```python
from build123d import *

# Parameters (mm, degrees)
F0_W     = 25.4
F0_H     = 25.4
F1_DEPTH = 304.8
F2_R     = 3.175
F3_DEPTH = 50.8
F4_R     = 3.175
F5_DEPTH = 25.4
F6_R     = 3.175
F7_DEPTH = 25.4
F8_DEPTH = 12.7


with BuildPart() as f1:
    # F0 (on Top) → F1 (new body)
    with BuildSketch(Plane.XY):
        Rectangle(F0_W, F0_H)
    extrude(amount=F1_DEPTH)

    # F2 (on face) → F3 (cut)
    with BuildSketch(Plane.XZ.offset(12.7)):
        with Locations((0, 292.1)):
            Circle(F2_R)
    extrude(amount=-F3_DEPTH, mode=Mode.SUBTRACT)

    # F4 (on face) → F5 (cut)
    with BuildSketch(Plane.YZ.offset(12.7)):
        with Locations((0, 292.1)):
            Circle(F4_R)
    extrude(amount=-F5_DEPTH, mode=Mode.SUBTRACT)

    # F6 (on face) → F7 (cut)
    with BuildSketch(Plane.YZ.offset(12.7)):
        with Locations((0, 4.7888585575)):
            Circle(F6_R)
    extrude(amount=-F7_DEPTH, mode=Mode.SUBTRACT)

    # F8 (add): a face of the model
    f8_faces = [f1.faces().sort_by_distance(p)[0] for p in [
        (0, 0, 0),
    ]]
    extrude(f8_faces, amount=F8_DEPTH)


solid = f1.part
```
Model file for the job. Use its own axes, mm. Give positions to 0.01 mm unless a question says otherwise; leave off trailing zeros. Order: outer loops, then holes, each group sorted by start corner. A loop starts at its lowest first (then second) coordinate and runs counter-clockwise, first axis right, second up.
1) Mould opens along Z. For faces 1 (the flat face through (12.7, 0, 148)), 2 (the cylindrical face through (3.03, -7.85, 293.05)), 3 (the flat face through (0, 0, -12.7)) say: +Z half, -Z half, draft (parallel to the pull), parting line (faces both ways), or undercut.
2) Wall check: probe 1 along Z at (x, y) = (5.5, 0) (3 decimals); probe 2 along Z at (x, y) = (-3.5, 0.5); probe 3 along Y at (x, z) = (-7.5, 292.1) (3 decimals). Give the ranges that are in metal, low to high.
3) Saw through at A-A, the plane z = 292.1. Write the cut outline in (x, y) (3 decimals), then the cut area to 3 significant figures.
Computed:
1. face 1: draft
1. face 2: undercut
1. face 3: -Z half
2. probe 1: z = -12.7 to 1.614, 7.964 to 288.925, 295.275 to 304.8
2. probe 2: z = -12.7 to 1.65, 7.92 to 288.96, 295.24 to 304.8
2. probe 3: y = -12.7 to -3.175, 3.175 to 12.7
3. outline: (-12.7, -12.7) - (-3.175, -12.7) - (-3.175, -3.175) - (-12.7, -3.175) - close; (-12.7, 3.175) - (-3.175, 3.175) - (-3.175, 12.7) - (-12.7, 12.7) - close; (3.175, -12.7) - (12.7, -12.7) - (12.7, -3.175) - (3.175, -3.175) - close; (3.175, 3.175) - (12.7, 3.175) - (12.7, 12.7) - (3.175, 12.7) - close
3. area: 363 mm2
